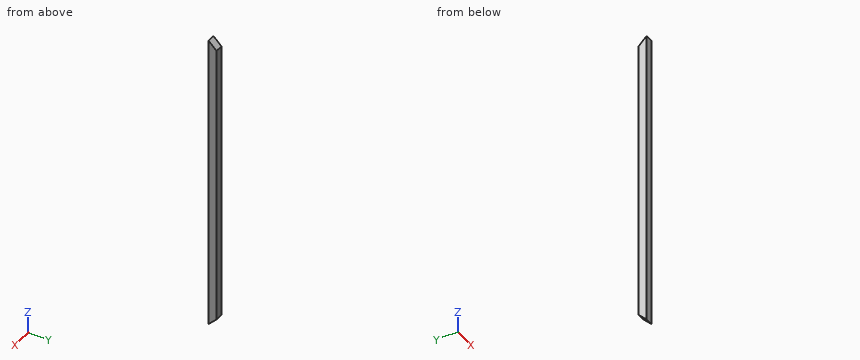
Autodesk Inventor part; units mm, degrees
ref_plane "YZ Plane" through (0, 0, 0) normal (1, 0, 0) x (0, 1, 0)
ref_plane "XZ Plane" through (0, 0, 0) normal (0, 1, 0) x (-1, 0, 0)
ref_plane "XY Plane" through (0, 0, 0) normal (0, 0, 1) x (1, 0, 0)
sketch "Sketch1" plane through (0, 0, 0) normal (0, 1, 0) x (-1, 0, 0)
  line L0 (0, 0) -> (-6.35, 0)
  line L1 (-6.35, 0) -> (-6.35, -244)
  line L2 (-6.35, -244) -> (0, -244)
  line L3 (0, -244) -> (0, 0)
  dimension "d0" = 6.35
  dimension "d1" = 244
extrude "Extrusion1" add sketch "Sketch1" along normal blind 6.35
sketch "Sketch2" plane through (6.35, 0, 0) normal (1, 0, 0) x (0, 0, -1)
  line L0 (0, 0) -> (244, 0)
  line L1 (0, 0) -> (6.35, 6.35)
  line L2 (0, 6.35) -> (244, 6.35)
  line L3 (0, 0) -> (8.9803, 0) construction
  line L4 (6.35, 6.35) -> (0, 6.35)
  line L5 (0, 6.35) -> (0, 0)
  dimension "d4" = 45
extrude "Extrusion2" cut sketch "Sketch2" against normal blind 10
sketch "Sketch3" plane through (6.35, 0, -244) normal (1, 0, 0) x (0, 0, -1)
  line L0 (0, 0) -> (-6.35, 6.35)
  line L1 (0, 6.35) -> (-237.65, 6.35)
  line L2 (0, 0) -> (8.9803, 0) construction
  line L3 (-6.35, 6.35) -> (0, 6.35)
  line L4 (0, 6.35) -> (0, 0)
  point P0 (-244, 0)
  dimension "d7" = 135
extrude "Extrusion3" cut sketch "Sketch3" against normal blind 10
properties part number "6"
The model under review builds one solid part; all positions refer to its coordinate system, in mm. Round coordinates to 2 decimals unless told otherwise and drop trailing zeros. Loops run counter-clockwise (first coordinate to the right, second up) from the corner with the lowest first, then second, coordinate; pieces in that order, holes last. Notation, with made-up numbers: (73.25, -18) -> (103.25, -18) arc R12 cw to (103.25, -13) -> close; hole circle Ø9 at (14, -3). An arc over 180 degrees is marked (long way). Answer as CSV lines item,"result".
1) For P1, Ø1, axis at x = 0.5, y = 3.5, coming from the +Z side; P2, Ø3, axis at y = 1.5, z = -147, coming from the -X side; P3, Ø2, axis at x = 3.5, y = 5.5, coming from the -Z side, all flat-tipped, find the tip position at first contact; note any pin that passes through.
Geometry results:
P1,"stops at z = -3"
P2,"stops at x = 0"
P3,"stops at z = -239.5"
2) Add section A-A on y = 5. Write out the cut boundary in (x, z), plus the area to 3 significant figures.
Geometry results:
outline,"(0, -239) -> (6.35, -239) -> (6.35, -5) -> (0, -5) -> close"
area,"1,490 mm²"
3) Add section B-B on x = 4. Write out the cut boundary in (y, z).
Geometry results:
outline,"(0, -244) -> (6.35, -237.65) -> (6.35, -6.35) -> (0, 0) -> close"
4) To check wall thickness, follow line 1 along Z through (x, y) = (1, 1.25); line 2 along Z through (x, y) = (5.25, 5). State the ranges of each line that lie inside material, in increasing order. Write a range as from..to.
Geometry results:
line 1,"z = -242.75..-1.25"
line 2,"z = -239..-5"
